For this review, take the finished solid that the model builds, in its own axes (mm). A direction names the side the tool comes from. Round coordinates to 2 decimals unless told otherwise and drop trailing zeros. Write each loop counter-clockwise with the first axis right and the second up, starting at its lowest first coordinate (ties: lowest second). Pieces come first, ordered by that corner, then holes. Notation, with made-up numbers: (-35.5, 39) - (11.5, 39) arc R36 ccw to (11.5, 78) - close; hole circle Ø6 at (-6.5, -5). An arc over 180 degrees is marked (long way). Answer in a Markdown table with one row per item. Add a question column.
Autodesk Inventor part; units mm, degrees
ref_plane "YZ Plane" through (0, 0, 0) normal (1, 0, 0) x (0, 1, 0)
ref_plane "XZ Plane" through (0, 0, 0) normal (0, 1, 0) x (-1, 0, 0)
ref_plane "XY Plane" through (0, 0, 0) normal (0, 0, 1) x (1, 0, 0)
sketch "Sketch1" plane through (0, 0, 0) normal (0, 0, 1) x (1, 0, 0)
  line L0 (0, 0) -> (50.8, 0)
  line L1 (50.8, 0) -> (50.8, 45.212)
  line L2 (50.8, 45.212) -> (0, 45.212)
  line L3 (0, 45.212) -> (0, 0)
  dimension "d0" = 50.8
  dimension "d1" = 45.212
extrude "Extrusion1" add sketch "Sketch1" along normal blind 3.175
sketch "Sketch3" plane through (0, 0, 3.175) normal (0, 0, 1) x (1, 0, 0)
  point P0 (0, 0)
sketch "Sketch4" plane through (0, 0, 3.175) normal (0, 0, 1) x (1, 0, 0)
  point P0 (0, 0)
sketch "Sketch5" plane through (0, 0, 3.175) normal (0, 0, 1) x (1, 0, 0)
  line L0 (6.35, 21.0058) -> (9.525, 21.0058)
  line L1 (9.525, 21.0058) -> (9.525, 24.1808)
  line L2 (9.525, 24.1808) -> (6.35, 24.1808)
  line L3 (6.35, 24.1808) -> (6.35, 21.0058)
  point P0 (0, 0)
  dimension "d12" = 3.175
  dimension "d13" = 3.175
extrude "Extrusion3" add sketch "Sketch5" along normal blind 6.35
hole "Hole1" at (7.9248, 21.0058, 7.9248) direction (0, 1, 0) diameter 1.27 end through all
properties part number "HingePart1MK2"
Q1. Draft analysis for pull direction Z (two halves, no side actions). For faces 6 (the face through (8, 23, 9.525)), 7 (the face through (50.8, 22, 2)), 8 (the face through (7.496, 22.616, 8.393)), state which applies: released by +Z, released by -Z, zero draft, split by the parting line, or undercut.
Q2. Insertion check: pin 1 Ø4 at (y, z) = (20, 4) entering from +X; pin 2 Ø22.5 at (x, y) = (27.5, 18) entering from +Z (3 decimals); pin 3 Ø1.6 at (y, z) = (22, 5) entering from +X (3 decimals); pin 4 Ø2.5 at (x, z) = (8.5, 6) entering from +Y. Each pin has a flat end and moves straight along its axis. Give the tip position at first contact, or say it passes through.
Q3. Add section B-B on z = 6.5. State the section outline as (x, y) points (3 decimals).
Q4. To check wall thickness, follow probe 1 along Z at (x, y) = (28, 3.5) (3 decimals); probe 2 along X at (y, z) = (24, 6.75) (3 decimals). State the ranges of each line that lie inside material, in increasing order.
Q5. Add section A-A on y = 37. State the section outline as (x, z) points (3 decimals), then the cut area to 3 significant figures.
Q6. Tool access review of faces 1 (the face through (8, 21.006, 6)), 2 (the face through (9.525, 23, 6)), 3 (the face through (6.35, 23, 6)), 4 (the face through (8, 24.181, 6)), 5 (the face through (25, 23, 0)): name each direction out of +Z, -Z, +X, -X, +Y, -Y from which nothing blocks a thin tool from reaching the whole face with its end or side.
Answer sheet:
| question | item | result |
|---|---|---|
| 1 | face 6 | released by +Z |
| 1 | face 7 | zero draft |
| 1 | face 8 | undercut |
| 2 | pin 1 | stops at x = 50.8 |
| 2 | pin 2 | stops at z = 3.175 |
| 2 | pin 3 | stops at x = 9.525 |
| 2 | pin 4 | stops at y = 24.18 |
| 3 | outline | (6.35, 21.006) - (9.525, 21.006) - (9.525, 24.181) - (6.35, 24.181) - close |
| 4 | probe 1 | z = 0 to 3.175 |
| 4 | probe 2 | x = 6.35 to 9.525 |
| 5 | outline | (0, 0) - (50.8, 0) - (50.8, 3.175) - (0, 3.175) - close |
| 5 | area | 161 mm² |
| 6 | face 1 | +Z, +X, -X, -Y |
| 6 | face 2 | +Z, +X, +Y, -Y |
| 6 | face 3 | +Z, -X, +Y, -Y |
| 6 | face 4 | +Z, +X, -X, +Y |
| 6 | face 5 | -Z, +X, -X, +Y, -Y |
